Check sheet for the modelled part. Datum: model origin and axes. Units: mm. Face numbers are marked on the shaded views. Round coordinates to 2 decimals unless told otherwise and drop trailing zeros. Write each loop counter-clockwise with the first axis right and the second up, starting at its lowest first coordinate (ties: lowest second). Pieces come first, ordered by that corner, then holes. Notation, with made-up numbers: (1, 72.25) -> (43, 72.25) arc R9 cw to (43, 85.25) -> close; hole circle Ø10 at (-38, 11.5). An arc over 180 degrees is marked (long way). Put each result on its own line as item: value. Start each with the question number.
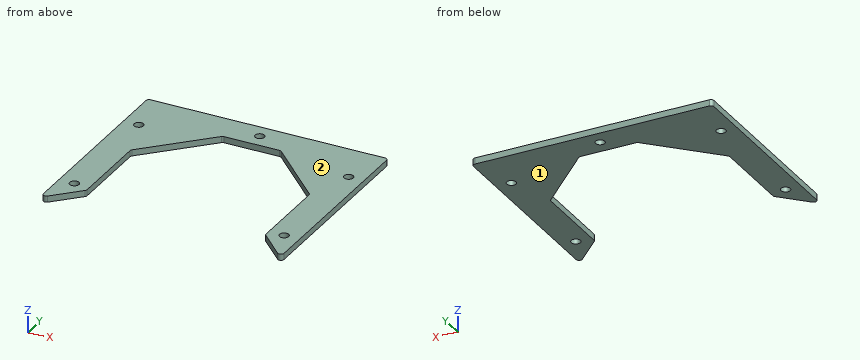
from build123d import *

# Parameters (mm, degrees)
SKETCH_R  = 3
PAD_DEPTH = 4


with BuildPart() as part:
    # Sketch → Pad (new body)
    with BuildSketch(Plane.XY):
        with BuildLine():
            Line((-78, 8), (-78, -119.313708))
            ThreePointArc((-78, -119.313708), (-76.765367, -121.161468), (-74.585786, -120.727922))
            Line((-74.585786, -120.727922), (-58.585786, -104.727922))
            ThreePointArc((-58.585786, -104.727922), (-58.152241, -104.079075), (-58, -103.313708))
            Line((-58, -50), (-58, -103.313708))
            ThreePointArc((-57.414214, -48.585786), (-57.847759, -49.234633), (-58, -50))
            Line((-57.414214, -48.585786), (-19.414214, -10.585786))
            ThreePointArc((-18, -10), (-18.765367, -10.152241), (-19.414214, -10.585786))
            Line((-18, -10), (18, -10))
            ThreePointArc((19.414214, -10.585786), (18.765367, -10.152241), (18, -10))
            Line((19.414214, -10.585786), (57.414214, -48.585786))
            ThreePointArc((58, -50), (57.847759, -49.234633), (57.414214, -48.585786))
            Line((58, -50), (58, -103.313708))
            ThreePointArc((58, -103.313708), (58.152241, -104.079075), (58.585786, -104.727922))
            Line((58.585786, -104.727922), (74.585786, -120.727922))
            ThreePointArc((74.585786, -120.727922), (76.765367, -121.161468), (78, -119.313708))
            Line((78, -119.313708), (78, 8))
            ThreePointArc((78, 8), (77.414214, 9.414214), (76, 10))
            Line((76, 10), (-76, 10))
            ThreePointArc((-76, 10), (-77.414214, 9.414214), (-78, 8))
        make_face()
        with Locations((-68, -20)):
            Circle(SKETCH_R, mode=Mode.SUBTRACT)
        with Locations((-68, -100)):
            Circle(SKETCH_R, mode=Mode.SUBTRACT)
        with Locations((68, -20)):
            Circle(SKETCH_R, mode=Mode.SUBTRACT)
        with Locations((68, -100)):
            Circle(SKETCH_R, mode=Mode.SUBTRACT)
        Circle(SKETCH_R, mode=Mode.SUBTRACT)
    extrude(amount=PAD_DEPTH)


solid = part.part
1. Draft check along Z on the marked faces 1 and 2. Enter one of: released by +Z, released by -Z, zero draft, split by the parting line, or undercut.
2. Section check A-A, the plane y = -100. Enter the section's corners in (x, z), then the cut area to 3 significant figures.
3. Material ranges on L1, parallel to X at y = -81.5, z = 1.1; L2, parallel to X at y = -99.5, z = 3.2; L3, parallel to Y at x = 70, z = 1.15, recorded low to high. Write a range as [from, to].
4. Gauge pin test, flat end, axial feed: P1, Ø2, axis at x = -9, z = 2, coming from the -Y side. Record the tip position at first contact, or that the pin passes through.
5. Section check C-C, the plane x = 0. Enter the section's corners in (y, z).
6. Section check D-D, the plane y = 0. Enter the section's corners in (x, z), then the cut area to 3 significant figures.
7. Section check B-B, the plane z = 1.8. Enter the section's corners in (x, y), then the cut area to 3 significant figures.
Reply:
1. face 1: released by -Z
1. face 2: released by +Z
2. outline: (-78, 0) -> (-71, 0) -> (-71, 4) -> (-78, 4) -> close; (-65, 0) -> (-58, 0) -> (-58, 4) -> (-65, 4) -> close; (58, 0) -> (65, 0) -> (65, 4) -> (58, 4) -> close; (71, 0) -> (78, 0) -> (78, 4) -> (71, 4) -> close
2. area: 112 mm2
3. L1: x = [-78, -58], [58, 78]
3. L2: x = [-78, -70.96], [-65.04, -58], [58, 65.04], [70.96, 78]
3. L3: y = [-116.14, -102.24], [-97.76, -22.24], [-17.76, 10]
4. P1: stops at y = -10
5. outline: (-10, 0) -> (-3, 0) -> (-3, 4) -> (-10, 4) -> close; (3, 0) -> (10, 0) -> (10, 4) -> (3, 4) -> close
6. outline: (-78, 0) -> (-3, 0) -> (-3, 4) -> (-78, 4) -> close; (3, 0) -> (78, 0) -> (78, 4) -> (3, 4) -> close
6. area: 600 mm2
7. outline: (-78, -119.31) arc R2 ccw to (-74.59, -120.73) -> (-58.59, -104.73) arc R2 ccw to (-58, -103.31) -> (-58, -50) arc R2 cw to (-57.41, -48.59) -> (-19.41, -10.59) arc R2 cw to (-18, -10) -> (18, -10) arc R2 cw to (19.41, -10.59) -> (57.41, -48.59) arc R2 cw to (58, -50) -> (58, -103.31) arc R2 ccw to (58.59, -104.73) -> (74.59, -120.73) arc R2 ccw to (78, -119.31) -> (78, 8) arc R2 ccw to (76, 10) -> (-76, 10) arc R2 ccw to (-78, 8) -> close; hole circle Ø6 at (-68, -100); hole circle Ø6 at (-68, -20); hole circle Ø6 at (0, 0); hole circle Ø6 at (68, -100); hole circle Ø6 at (68, -20)
7. area: 8,670 mm2
